```python
from build123d import *
from build123d.topology import SkipClean

# Parameters (mm, degrees)
SKETCH_1_R                  = 2
EXTRUDE_1_DEPTH             = 61.5
EXTRUDE_START               = -35
SKETCH_2_R                  = 2.5
EXTRUDE_2_DEPTH             = 1.5
SKETCH_3_R                  = 1.7
EXTRUDE_3_DEPTH             = 2
EXTRUDE_4_DEPTH             = 5
SKETCH_5_R                  = 2
EXTRUDE_5_DEPTH             = 4
EXTRUDE_6_DEPTH             = 2
EXTRUDE_6_DEPTH_BACK        = 2
CUT_EXTRUDE_1_REACH         = 72.721
SKETCH_8_R                  = 1.5
EXTRUDE_7_DEPTH             = 6.5
EXTRUDE_7_DIRECTION_2_REACH = 75.536
CHAMFER_1_SIZE              = 0.4
EXTRUDE_8_DEPTH             = 0.75
EXTRUDE_8_DEPTH_BACK        = 0.75


with BuildPart() as part:
    # Sketch 1 → Extrude 1 (new body)
    with BuildSketch(Plane.XY):
        Circle(SKETCH_1_R)
    extrude(amount=EXTRUDE_1_DEPTH)

    # Sketch 2 → Extrude 2 (add)
    with BuildSketch(Plane.XY.offset(61.5).offset(EXTRUDE_START)):
        Circle(SKETCH_2_R)
    extrude(amount=-EXTRUDE_2_DEPTH)

    # Sketch 3 → Extrude 3 (add)
    with BuildSketch(Plane.XY.offset(61.5)):
        Circle(SKETCH_3_R)
    extrude(amount=EXTRUDE_3_DEPTH)

    # Sketch 4 → Extrude 4 (add)
    with BuildSketch(Plane.XY.offset(63.5)):
        Polygon((0, 2), (-1.732050808, 1), (-1.732050808, -1), (0, -2), (1.732050808, -1), (1.732050808, 1), align=None)
    extrude(amount=EXTRUDE_4_DEPTH)



with BuildPart() as body_2:
    # Sketch 5 → Extrude 5 (new body)
    with BuildSketch(Plane(origin=(0, 0, 1), x_dir=(-1, 0, 0), z_dir=(0, 0, -1))):
        with Locations((-15, 0)):
            Circle(SKETCH_5_R)
    extrude(amount=EXTRUDE_5_DEPTH)


with BuildPart() as part_1:
    add(part.part)

    add(body_2.part)  # Extrude 6 merges body 2
    # Sketch 6 → Extrude 6 (add, two sides: drawn at the far end of the back side and taken through both)
    with BuildSketch(Plane(origin=(0, 0, 0), x_dir=(1, 0, 0), z_dir=(0, 1, 0)).offset(-EXTRUDE_6_DEPTH_BACK)):
        Polygon((0, 0), (15, 3), (15, -1), (0, -4), align=None)
    extrude(amount=EXTRUDE_6_DEPTH + EXTRUDE_6_DEPTH_BACK)

    # Sketch 7 → Cut-Extrude 1 (cut, up to next)
    with BuildSketch(Plane(origin=(0, 2, 0), x_dir=(1, 0, 0), z_dir=(0, 1, 0)), mode=Mode.PRIVATE) as cut_extrude_1_sk1:
        Polygon((0, 0), (-2, 0), (-2, -2.5), align=None)
    cut_extrude_1_tool1 = extrude(cut_extrude_1_sk1.sketch, amount=-CUT_EXTRUDE_1_REACH, mode=Mode.PRIVATE) & part_1.part
    # Sketch 7 → Cut-Extrude 1 (cut, up to next)
    with BuildSketch(Plane(origin=(0, 2, 0), x_dir=(1, 0, 0), z_dir=(0, 1, 0)), mode=Mode.PRIVATE) as cut_extrude_1_sk2:
        Polygon((15, -1), (17, 1.5), (17, -1), align=None)
    cut_extrude_1_tool2 = extrude(cut_extrude_1_sk2.sketch, amount=-CUT_EXTRUDE_1_REACH, mode=Mode.PRIVATE) & part_1.part
    # Sketch 7 → Cut-Extrude 1 (cut, up to next)
    with BuildSketch(Plane(origin=(0, 2, 0), x_dir=(1, 0, 0), z_dir=(0, 1, 0)), mode=Mode.PRIVATE) as cut_extrude_1_sk3:
        Polygon((15, 3), (13, 2.6), (13, 3), align=None)
    cut_extrude_1_tool3 = extrude(cut_extrude_1_sk3.sketch, amount=-CUT_EXTRUDE_1_REACH, mode=Mode.PRIVATE) & part_1.part
    add(cut_extrude_1_tool1.solids().sort_by_distance((-1.333333, 2, 0.833333))[0], mode=Mode.SUBTRACT)
    add(cut_extrude_1_tool2.solids().sort_by_distance((16.333333, 2, 0.166667))[0], mode=Mode.SUBTRACT)
    add(cut_extrude_1_tool3.solids().sort_by_distance((13.666667, 2, -2.866667))[0], mode=Mode.SUBTRACT)

    # Sketch 8 → Extrude 7 (add)
    with BuildSketch(Plane(origin=(0, 0, -3), x_dir=(-1, 0, 0), z_dir=(0, 0, -1))):
        with Locations((-15.4, 0)):
            Circle(SKETCH_8_R)
    extrude(amount=EXTRUDE_7_DEPTH)

    # Sketch 8 → Extrude 7 direction 2 (add, up to next)
    with BuildSketch(Plane(origin=(0, 0, -3), x_dir=(-1, 0, 0), z_dir=(0, 0, -1)), mode=Mode.PRIVATE) as extrude_7_direction_2_sk1:
        with Locations((-15.4, 0)):
            Circle(SKETCH_8_R)
    extrude_7_direction_2_tool1 = extrude(extrude_7_direction_2_sk1.sketch, amount=-EXTRUDE_7_DIRECTION_2_REACH, mode=Mode.PRIVATE) - part_1.part
    add(extrude_7_direction_2_tool1.solids().sort_by_distance((15.4, 0, -3))[0])

    # Sketch 9 → Revolve 1 (revolve)
    with SkipClean():  # the faces are left unmerged after this step: merging them gives an invalid solid
        with BuildSketch(Plane(origin=(0, 0, 0), x_dir=(1, 0, 0), z_dir=(0, 1, 0))):
            with BuildLine():
                Line((15.4, 9.5), (15.4, 7.5))
                Line((15.4, 7.5), (15.4, 5.5))
                ThreePointArc((15.4, 5.5), (17.4, 7.5), (15.4, 9.5))
            make_face()
        revolve(axis=Axis((15.4, 0, -9.5), (0, 0, 1)))
    add(part_1.part.scale(1), mode=Mode.REPLACE)  # the faces are merged on a copy

    # Chamfer 1
    chamfer_1_edges = [part_1.edges().sort_by_distance(p)[0] for p in [
        (16.9, 0, -9.5),
    ]]
    chamfer(chamfer_1_edges, length=CHAMFER_1_SIZE)

    # Sketch 10 → Extrude 8 (add, two sides: drawn at the far end of the back side and taken through both)
    with SkipClean():  # the faces are left unmerged after this step: merging them gives an invalid solid
        with BuildSketch(Plane(origin=(0, 0, 0), x_dir=(1, 0, 0), z_dir=(0, 1, 0)).offset(-EXTRUDE_8_DEPTH_BACK)):
            Polygon((0, -2), (0, -8), (6, -2.8), (8, -1.066666667), align=None)
        extrude(amount=EXTRUDE_8_DEPTH + EXTRUDE_8_DEPTH_BACK)


solid = part_1.part
```
CAD build for the part. Positions are in the model's coordinates, mm. A direction names the side the tool comes from. Coordinates: 2 decimals unless noted, no trailing zeros. Order: outer loops, then holes, each group sorted by start corner. A loop starts at its lowest first (then second) coordinate and runs counter-clockwise, first axis right, second up.
(1) Saw through at B-B, the plane x = -0.75. Write the cut outline in (y, z), and give its area (3 significant figures).
Solution:
outline: (-2.38, 25) - (-1.85, 25) - (-1.85, 0.94) - (1.85, 0.94) - (1.85, 25) - (2.38, 25) - (2.38, 26.5) - (1.85, 26.5) - (1.85, 61.5) - (1.53, 61.5) - (1.53, 63.5) - (1.57, 63.5) - (1.57, 68.5) - (-1.57, 68.5) - (-1.57, 63.5) - (-1.53, 63.5) - (-1.53, 61.5) - (-1.85, 61.5) - (-1.85, 26.5) - (-2.38, 26.5) - close
area: 248 mm2
(2) Mould opens along Z. For faces 5 (the face through (-0.37, -1.66, 62.49)), 6 (the face through (0.88, 1.49, 65.96)), 7 (the face through (0, 0, 68.5)), 8 (the face through (-0.8, 0, 1)) say: released by +Z, released by -Z, zero draft, split by the parting line, or undercut.
Solution:
face 5: undercut
face 6: zero draft
face 7: released by +Z
face 8: released by -Z
(3) Saw through at C-C, the plane x = 7. Write the cut outline in (y, z).
Solution:
outline: (-2, -1.4) - (2, -1.4) - (2, 2.6) - (-2, 2.6) - close
(4) Which spindle directions (+Z, -Z, +X, -X, +Y, -Y) get a long thin tool onto all of the face, cutting with end or side? Do faces 1 (the face through (-0.85, 1.51, 65.96)), 2 (the face through (0, -2, 44)), 3 (the face through (17, 0, -2)), 4 (the face through (-1.732, 0, 66)). Say none if no direction does.
Solution:
face 1: +Z, -X, +Y
face 2: +Z
face 3: +Z, +X
face 4: +Z, -X, +Y, -Y
(5) Drill centre lines: L1, parallel to Z at x = -0.5, y = 2.35; L2, parallel to Z at x = 1.75, y = 1.45; L3, parallel to Z at x = 3.5, y = -1.45. Where is each one in solid material? Low to high.
Solution:
L1: z = 25 to 26.5
L2: z = -0.35 to 3.65, 25 to 26.5
L3: z = -0.7 to 3.3
(6) Pin check, flat tips, straight feed: pin 1 Ø2 at (x, z) = (6.5, 1) entering from +Y; pin 2 Ø1 at (x, y) = (2, 0) entering from -Z; pin 3 Ø3 at (x, y) = (0, 0) entering from -Z. Stop position of each tip, or through.
Solution:
pin 1: stops at y = 2
pin 2: stops at z = -0.5
pin 3: stops at z = -0.3
(7) Saw through at A-A, the plane z = 52.5. Write the cut outline in (x, y), and give its area (3 significant figures).
Solution:
outline: circle Ø4 at (0, 0)
area: 12.6 mm2
